```python
from build123d import *

# Parameters (mm, degrees)
SKETCH_1_R          = 9.52
SKETCH_1_R_2        = 1.25
EXTRUDE_1_DEPTH     = 2
SKETCH_2_R          = 2.05
CUT_EXTRUDE_1_DEPTH = 4
FILLET_1_R          = 2
FILLET_3_R          = 30
FILLET_6_R          = 10


with BuildPart() as part:
    # 草图1 → 凸台-拉伸1 (new body)
    with BuildSketch(Plane.XY):
        with BuildLine():
            Line((328.542857143, -40.145714286), (-1.457142857, -40.145714286))
            Line((-1.457142857, -40.145714286), (-7.409980895, -22.36200829))
            ThreePointArc((-7.409980895, -22.36200829), (-24.457142857, -0.145714286), (-7.409980895, 22.070579719))
            Line((-7.409980895, 22.070579719), (-1.457142857, 39.854285714))
            Line((-1.457142857, 39.854285714), (75.684411109, 39.854285714))
            Line((75.684411109, 39.854285714), (85.544413109, 61.154285714))
            Line((85.544413109, 61.154285714), (96.174870529, 61.154285714))
            Line((96.174870529, 61.154285714), (106.145912956, 39.854285714))
            Line((106.145912956, 39.854285714), (321.071621128, 39.854285714))
            Line((321.071621128, 39.854285714), (328.542857143, 39.854285714))
            Line((328.542857143, 39.854285714), (334.49569518, 22.070579719))
            ThreePointArc((334.49569518, 22.070579719), (351.542857143, -0.145714286), (334.49569518, -22.36200829))
            Line((334.49569518, -22.36200829), (328.542857143, -40.145714286))
        make_face()
        with Locations((-1.457142857, -0.145714286)):
            Circle(SKETCH_1_R, mode=Mode.SUBTRACT)
        with Locations((328.542857143, -0.145714286)):
            Circle(SKETCH_1_R, mode=Mode.SUBTRACT)
        with Locations((318.542857143, 32.854285714)):
            Circle(SKETCH_1_R_2, mode=Mode.SUBTRACT)
        with BuildLine():
            ThreePointArc((318.542857143, 22.154285714), (326.108899702, 25.288243156), (329.242857143, 32.854285714))
            ThreePointArc((329.242857143, 32.854285714), (328.042857143, 34.054285714), (326.842857143, 32.854285714))
            ThreePointArc((326.842857143, 32.854285714), (324.411843427, 26.98529943), (318.542857143, 24.554285714))
            ThreePointArc((318.542857143, 24.554285714), (317.342857143, 23.354285714), (318.542857143, 22.154285714))
        make_face(mode=Mode.SUBTRACT)
    extrude(amount=EXTRUDE_1_DEPTH)

    # 草图2 → 切除-拉伸1 (cut)
    with BuildSketch(Plane.XY.offset(2)):
        with Locations((108.542857143, 33.854285714)):
            Circle(SKETCH_2_R)
        with Locations((198.542857143, 33.854285714)):
            Circle(SKETCH_2_R)
        with Locations((288.542857143, 33.854285714)):
            Circle(SKETCH_2_R)
        with Locations((108.542857143, -34.145714286)):
            Circle(SKETCH_2_R)
        with Locations((198.542857143, -34.145714286)):
            Circle(SKETCH_2_R)
        with Locations((288.542857143, -34.145714286)):
            Circle(SKETCH_2_R)
        with Locations((18.542857143, -34.145714286)):
            Circle(SKETCH_2_R)
        with Locations((18.542857143, 33.854285714)):
            Circle(SKETCH_2_R)
        Polygon((31.542857143, -21.145714286), (104.183898028, -21.145714286), (159.772133322, 20.854285714), (31.542857143, 20.854285714), align=None)
        Polygon((147.313580964, -21.145714286), (202.901816258, 20.854285714), (282.737923896, 20.854285714), (301.563806249, -0.145714286), (282.737923896, -21.145714286), align=None)
    extrude(amount=-CUT_EXTRUDE_1_DEPTH, mode=Mode.SUBTRACT)

    # 圆角1
    fillet_1_edges = [part.edges().sort_by_distance(p)[0] for p in [
        (202.901816258, 20.854285714, 1),
        (282.737923896, 20.854285714, 1),
        (301.563806249, -0.145714286, 1),
        (31.542857143, -21.145714286, 1),
        (31.542857143, 20.854285714, 1),
        (159.772133322, 20.854285714, 1),
        (104.183898028, -21.145714286, 1),
        (282.737923896, -21.145714286, 1),
        (147.313580964, -21.145714286, 1),
    ]]
    fillet(fillet_1_edges, radius=FILLET_1_R)

    # 圆角3
    # the kernel refuses this fillet: 30 mm, written as the material it takes off along each edge
    with BuildSketch(Plane(origin=(328.542857143, -40.145714286, -53.618003483), x_dir=(0.3174242162824087, 0.9482836426499714, 0), z_dir=(0, 0, 1))) as fillet_3_piece_1:
        with BuildLine():
            CenterArc((21.640648186, 29.86075675), FILLET_3_R, 198.507223716, 65.970321092)
            Line((-6.807861094, 20.338030262), (-7.376831279, 20.147575732))
            Line((-7.376831279, 20.147575732), (-0.568970186, -0.19045453))
            Line((-0.568970186, -0.19045453), (0, -0.6))
            ThreePointArc((0, -0.6), (9.376786225, -0.6), (18.695830935, -0.597215135))
            Line((18.695830935, -0.597215135), (18.75357245, 0))
        make_face()
    extrude(amount=109.236006966, mode=Mode.SUBTRACT)

    # 圆角6
    fillet_6_edges = [part.edges().sort_by_distance(p)[0] for p in [
        (328.542857143, 39.854285714, 1),
    ]]
    fillet(fillet_6_edges, radius=FILLET_6_R)


solid = part.part
```
The listing builds one solid part. Answer for the finished solid, in the listing's coordinates (mm). A direction names the side the tool comes from. Give positions to 0.01 mm unless a question says otherwise; leave off trailing zeros. Order: outer loops, then holes, each group sorted by start corner. A loop starts at its lowest first (then second) coordinate and runs counter-clockwise, first axis right, second up. Notation, with made-up numbers: (70.25, -21.75) -> (98.25, -21.75) arc R26 cw to (98.25, 3.25) -> close; hole circle Ø1 at (86.25, 54.25). An arc over 180 degrees is marked (long way). Answer as CSV lines item,"result". Start each with the question number.
Q1. Find the intervals of material crossed by L1, parallel to Y at x = 67.5, z = 0.7; L2, parallel to X at y = 8, z = 0.6; L3, parallel to X at y = -17, z = 0.7, in increasing order.
Q2. A cutting plane is placed at C-C (x = 120). Determine the outline of the cut face in (y, z).
Q3. A cutting plane is placed at A-A (x = 51). Determine the outline of the cut face in (y, z).
Q4. A cutting plane is placed at B-B (z = 1.5). Count the separate pieces of the cut face and the enclosed holes in it, then the cut area to 3 significant figures.
Q5. Determine the mould class of faces 1 (the cylindrical face through (351.54, 0.28, 0.99)), 2 (the flat face through (-4.475, 30.838, 0.986)), 3 (the cylindrical face through (324.476, 27.05, 0.986)), 4 (the flat face through (291.731, 10.822, 1.014)) for opening direction X: pulls with the +X half, pulls with the -X half, needs draft (parallel to the pull), parting line crosses it, or undercut.
Q6. A cutting plane is placed at D-D (y = 45). Determine the outline of the cut face in (x, z).
Q7. Which of the six approach directions +Z, -Z, +X, -X, +Y, -Y give full straight-line access (tool end or side, diameter ignored) to faces 5 (the flat face through (176.868, 1.184, 1.014)), 6 (the cylindrical face through (323.225, -35.441, 0.986))?
Q8. Given pin 1 (0.6 mm diameter, centred on x = 27.5, z = 1, fed in from +Y), flat-ended and moving along its own axis, determine where the tip first touches the part or whether it passes through.
Results found:
1,L1,"-40.15 to -21.15, 20.85 to 39.85"
1,L2,"-22.97 to -6.38, 3.47 to 31.54, 142.76 to 185.89, 294.26 to 323.62, 333.47 to 350.05"
1,L3,"-17.11 to 31.54, 109.67 to 152.8, 286.45 to 344.19"
2,outline,"(-40.15, 0) -> (-9.2, 0) -> (-9.2, 2) -> (-40.15, 2) -> close; (20.85, 0) -> (39.85, 0) -> (39.85, 2) -> (20.85, 2) -> close"
3,outline,"(-40.15, 0) -> (-21.15, 0) -> (-21.15, 2) -> (-40.15, 2) -> close; (20.85, 0) -> (39.85, 0) -> (39.85, 2) -> (20.85, 2) -> close"
4,separate pieces,"1"
4,enclosed holes,"14"
4,area,"18,800 mm2"
5,face 1,"pulls with the +X half"
5,face 2,"pulls with the -X half"
5,face 3,"undercut"
5,face 4,"undercut"
6,outline,"(78.07, 0) -> (103.74, 0) -> (103.74, 2) -> (78.07, 2) -> close"
7,face 5,"+Z, -Z"
7,face 6,"+Z, -Z, +X, -Y"
8,pin 1,"y = 39.85"
